The listing builds one solid part. Answer for the finished solid, in the listing's coordinates (mm). Face numbers are marked on the shaded views. A direction names the side the tool comes from. Round coordinates to 2 decimals unless told otherwise and drop trailing zeros. Loops run counter-clockwise (first coordinate to the right, second up) from the corner with the lowest first, then second, coordinate; pieces in that order, holes last. Notation, with made-up numbers: M -31,66 L -22,66 A10 ccw -22,70 Z; hole C 9,-25.5 d7. An arc over 180 degrees is marked long. Put each result on its own line as item: value. Start each with the question number.
(1) Section B-B, the plane z = 3.25 is taken. Determine the outline of the cut face in (x, y).
(2) Determine the mould class of the marked faces 3, 4 and 5 for opening direction Y: released by +Y, released by -Y, zero draft, split by the parting line, or undercut.
(3) Section A-A, the plane x = -5 is taken. Determine the outline of the cut face in (y, z), then the cut area to 3 significant figures.
(4) Section C-C, the plane y = -19 is taken. Determine the outline of the cut face in (x, z), then the cut area to 3 significant figures.
(5) Flat-ended cylindrical pins translate along their axes: P1, Ø6.5, axis at y = -16, z = 3.5, coming from the -X side; P2, Ø0.6, axis at x = -21.5, y = -23, coming from the -Z side; P3, Ø0.8, axis at x = -0.5, z = 13, coming from the -Y side. Find the tip coordinate at first contact, or state that the pin passes through.
(6) Straight lines are drawn through the part: line 1 (X direction, y = -22.25, z = 5.25); line 2 (Y direction, x = -28.5, z = 6.5); line 3 (X direction, y = -4.75, z = 3.25). For each, find the intervals that lie inside material, in ascending order.
(7) Section D-D, the plane z = -6.75 is taken. Determine the outline of the cut face in (x, y).
(8) Which of the six approach directions +Z, -Z, +X, -X, +Y, -Y give full straight-line access (tool end or side, diameter ignored) to the marked faces 1 and 2?
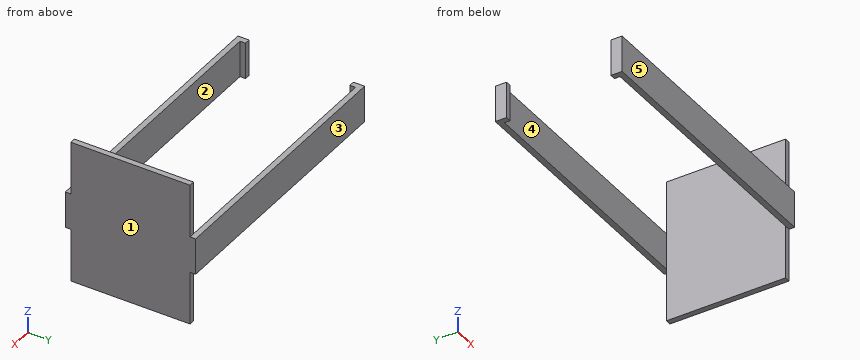
```python
from build123d import *

# Parameters (mm, degrees)
F0_W       = 46.99
F0_H       = 6.604
F1_DEPTH   = 1.016
F2_W       = 0.508
F2_H       = 6.604
F2_W_2     = 1.016
F3_DEPTH   = 1.016
F4_W       = 1.016
F4_H       = 6.604
F5_DEPTH   = 1.016
F6_W       = 1.016
F6_H       = 6.604
F7_DEPTH   = 21.59
F7_FACE_W  = 1.016
F7_FACE_H  = 6.604
F8_DEPTH   = 1.016
F9_W       = 1.016
F9_H       = 6.604
F10_DEPTH  = 46.99
F10_FACE_W = 1.016
F10_FACE_H = 6.604
F11_DEPTH  = 1.524
F12_W      = 1.016
F12_H      = 6.604
F13_DEPTH  = 1.016
F14_W      = 1.016
F14_H      = 21.59
F16_DEPTH  = 9.652
F17_W      = 1.016
F17_H      = 21.59
F18_DEPTH  = 9.652


with BuildPart() as f1:
    # F0 (on Front) → F1 (new body)
    with BuildSketch(Plane.XZ):
        with Locations((-23.495, 3.302)):
            Rectangle(F0_W, F0_H)
    extrude(amount=F1_DEPTH)

    # F2 (on face) → F3 (join)
    with BuildSketch(Plane.XZ.offset(1.016)):
        with Locations((-47.244, 3.302)):
            Rectangle(F2_W, F2_H)
        with Locations((-48.006, 3.302)):
            Rectangle(F2_W_2, F2_H)
    extrude(amount=-F3_DEPTH)

    # F4 (on face) → F5 (join)
    with BuildSketch(Plane.XZ.offset(1.016)):
        with Locations((-48.006, 3.302)):
            Rectangle(F4_W, F4_H)
    extrude(amount=F5_DEPTH)

    # F6 (on face) → F7 (join)
    with BuildSketch(Plane.XZ.offset(1.016)):
        with Locations((-0.508, 3.302)):
            Rectangle(F6_W, F6_H)
    extrude(amount=F7_DEPTH)

    # F7_face (on face) → F8 (join)
    with BuildSketch(Plane(origin=(-0.508, -22.606, 3.302), x_dir=(1, 0, 0), z_dir=(0, -1, 0))):
        Rectangle(F7_FACE_W, F7_FACE_H)
    extrude(amount=F8_DEPTH)

    # F9 (on face) → F10 (join)
    with BuildSketch(Plane(origin=(-1.016, 0, 0), x_dir=(0, -1, 0), z_dir=(-1, 0, 0))):
        with Locations((23.114, 3.302)):
            Rectangle(F9_W, F9_H)
    extrude(amount=F10_DEPTH)

    # F10_face (on face) → F11 (join)
    with BuildSketch(Plane(origin=(-48.006, -23.114, 3.302), x_dir=(0, -1, 0), z_dir=(-1, 0, 0))):
        Rectangle(F10_FACE_W, F10_FACE_H)
    extrude(amount=F11_DEPTH)

    # F12 (on face) → F13 (join)
    with BuildSketch(Plane(origin=(0, -22.606, 0), x_dir=(-1, 0, 0), z_dir=(0, 1, 0))):
        with Locations((49.022, 3.302)):
            Rectangle(F12_W, F12_H)
    extrude(amount=F13_DEPTH)

    # F14 (on face) → F16 (join)
    with BuildSketch(Plane.XY.offset(6.604)):
        with Locations((-0.508, -11.811)):
            Rectangle(F14_W, F14_H)
    extrude(amount=F16_DEPTH)

    # F17 (on face) → F18 (join)
    with BuildSketch(Plane(origin=(0, 0, 0), x_dir=(1, 0, 0), z_dir=(0, 0, -1))):
        with Locations((-0.508, 11.811)):
            Rectangle(F17_W, F17_H)
    extrude(amount=F18_DEPTH)


solid = f1.part
```
Recorded:
1. outline: M -49.53,-23.62 L 0,-23.62 L 0,0 L -48.51,0 L -48.51,-2.03 L -47.5,-2.03 L -47.5,-1.02 L -1.02,-1.02 L -1.02,-22.61 L -48.51,-22.61 L -48.51,-21.59 L -49.53,-21.59 Z
2. face 3: released by +Y
2. face 4: undercut
2. face 5: released by -Y
3. outline: M -23.62,0 L -22.61,0 L -22.61,6.6 L -23.62,6.6 Z; M -1.02,0 L 0,0 L 0,6.6 L -1.02,6.6 Z
3. area: 13.4 mm²
4. outline: M -1.02,-9.65 L 0,-9.65 L 0,16.26 L -1.02,16.26 Z
4. area: 26.3 mm²
5. P1: stops at x = -1.02
5. P2: stops at z = 0
5. P3: stops at y = -22.61
6. line 1: x = -49.53 to -48.51, -1.02 to 0
6. line 2: y = -23.62 to -22.61, -1.02 to 0
6. line 3: x = -1.02 to 0
7. outline: M -1.02,-22.61 L 0,-22.61 L 0,-1.02 L -1.02,-1.02 Z
8. face 1: +Z, -Z, +X, +Y, -Y
8. face 2: +Z, -Z
